Input: dimensioned drawing with shaded views. Units: mm. Origin: part minimum x, y, z. A direction names the side the tool comes from. Give positions to 0.01 mm unless a question says otherwise; leave off trailing zeros. Loops run counter-clockwise (first coordinate to the right, second up) from the corner with the lowest first, then second, coordinate; pieces in that order, holes last.
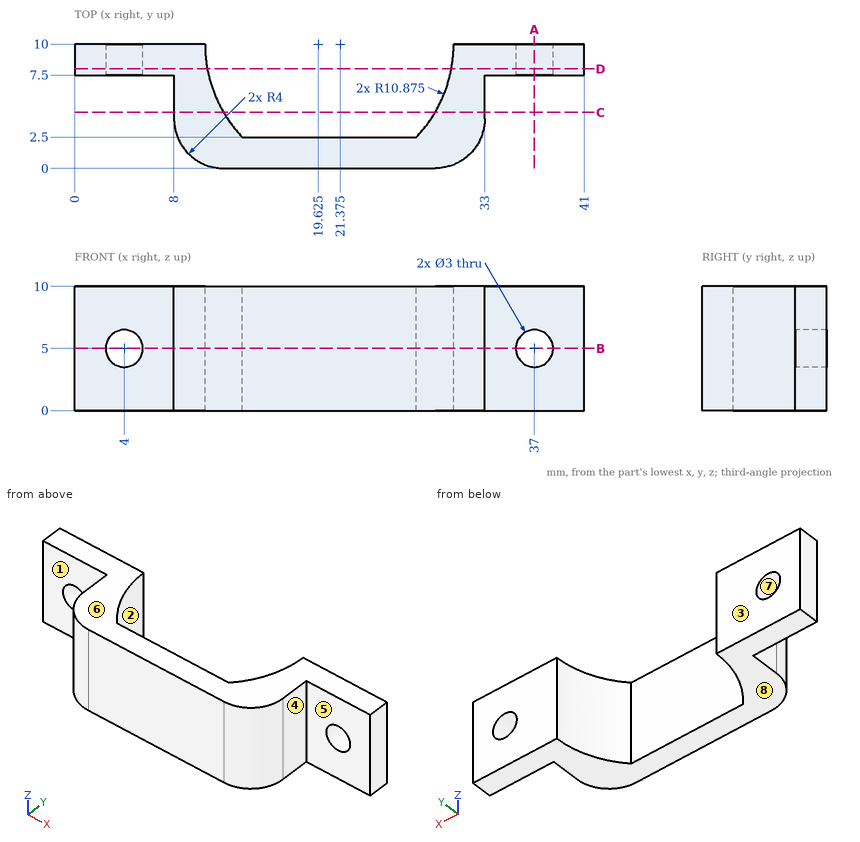
Item 1: Ray query, probe 1 along Z at (x, y) = (37, 8.3); probe 2 along X at (y, z) = (4.75, 4.75); probe 3 along Y at (x, z) = (19.5, 8). Return the intervals inside material, ascending.
Values follow:
probe 1: z = 0 to 3.5, 6.5 to 10
probe 2: x = 8 to 11.85, 29.15 to 33
probe 3: y = 0 to 2.5
Item 2: Section query D-D on y = 8. Return loops of the section in (x, z), plus the area to 3 significant figures.
Values follow:
outline: (0, 0) - (10.69, 0) - (10.69, 10) - (0, 10) - close; (30.31, 0) - (41, 0) - (41, 10) - (30.31, 10) - close; hole circle Ø3 at (4, 5); hole circle Ø3 at (37, 5)
area: 200 mm2
Item 3: Draft query along Z for the marked faces 5, 6, 7 and 8. Return one class per face: +Z half, -Z half, draft (parallel to the pull), parting line (faces both ways), or undercut.
Values follow:
face 5: draft
face 6: +Z half
face 7: undercut
face 8: -Z half
Item 4: Section query C-C on y = 4.5. Return loops of the section in (x, z).
Values follow:
outline: (8, 0) - (11.99, 0) - (11.99, 10) - (8, 10) - close; (29.01, 0) - (33, 0) - (33, 10) - (29.01, 10) - close
Item 5: Section query A-A on x = 37. Return loops of the section in (y, z), plus the area to 3 significant figures.
Values follow:
outline: (7.5, 0) - (10, 0) - (10, 3.5) - (7.5, 3.5) - close; (7.5, 6.5) - (10, 6.5) - (10, 10) - (7.5, 10) - close
area: 17.5 mm2
Item 6: Section query B-B on z = 5. Return loops of the section in (x, y) (3 decimals), plus the area to 3 significant figures.
Values follow:
outline: (0, 7.5) - (2.5, 7.5) - (2.5, 10) - (0, 10) - close; (5.5, 7.5) - (8, 7.5) - (8, 4) arc R4 ccw to (12, 0) - (29, 0) arc R4 ccw to (33, 4) - (33, 7.5) - (35.5, 7.5) - (35.5, 10) - (30.5, 10) arc R10.875 cw to (27.5, 2.5) - (13.5, 2.5) arc R10.875 cw to (10.5, 10) - (5.5, 10) - close; (38.5, 7.5) - (41, 7.5) - (41, 10) - (38.5, 10) - close
area: 132 mm2
Item 7: Set-up query: the marked faces 1, 2, 3 and 4. Return all of +Z, -Z, +X, -X, +Y, -Y with unobstructed straight access to the full face (end or side cutting, diameter ignored); none if empty.
Values follow:
face 1: +Z, -Z, -X, -Y
face 2: +Z, -Z, +Y
face 3: +Z, -Z, +X, -X, +Y
face 4: +Z, -Z, +X, -Y
Item 8: Pin query (flat end, axial travel): pin 1 (5 mm diameter, centred on x = 4, z = 5, fed in from -Y); pin 2 (3 mm diameter, centred on y = 5.5, z = 6.5, fed in from -X); pin 3 (1.5 mm diameter, centred on y = 6.5, z = 8.5, fed in from +X). Return the tip coordinate at first contact, or that it passes through.
Values follow:
pin 1: stops at y = 7.5
pin 2: stops at x = 8
pin 3: stops at x = 33
